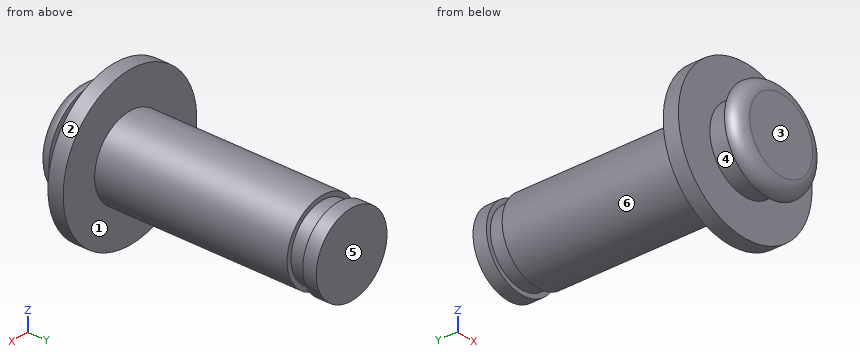
```python
from build123d import *


with BuildPart() as part:
    # Esboço1 → Revolução1 (revolve)
    with BuildSketch(Plane(origin=(0, 0, 0), x_dir=(0, 0, -1), z_dir=(1, 0, 0)), mode=Mode.PRIVATE) as revolu_o1_sk:
        with BuildLine():
            Line((0, 30.4), (0, 0))
            Line((0, 0), (-4, 0))
            ThreePointArc((-4, 0), (-5.060660172, 0.439339828), (-5.5, 1.5))
            Line((-5.5, 1.5), (-4.5, 1.5))
            Line((-4.5, 1.5), (-4.5, 4))
            Line((-4.5, 4), (-8.5, 4))
            Line((-8.5, 4), (-8.5, 5.7))
            Line((-8.5, 5.7), (-4.5, 5.7))
            Line((-4.5, 5.7), (-4.5, 27.15))
            Line((-4.5, 27.15), (-4, 27.15))
            Line((-4, 27.15), (-4, 28.9))
            Line((-4, 28.9), (-4.5, 28.9))
            Line((-4.5, 28.9), (-4.5, 30.4))
            Line((-4.5, 30.4), (0, 30.4))
        make_face()
    revolve(revolu_o1_sk.sketch.rotate(Axis((0, 0, 0), (0, 1, 0)), 180), axis=Axis((0, 0, 0), (0, 1, 0)))


solid = part.part
```
Could you check a few things on this model? Use its own coordinates, in mm. Face numbers are marked on the shaded views. A direction names the side the tool comes from. Coordinates: 2 decimals unless noted, no trailing zeros. Order: outer loops, then holes, each group sorted by start corner. A loop starts at its lowest first (then second) coordinate and runs counter-clockwise, first axis right, second up. Notation, with made-up numbers: M 68.25,89 L 124.25,89 A15 ccw 124.25,113 Z; hole C 89.5,85 d5. An arc over 180 degrees is marked long. Use a Markdown table: item, result. Add a question column.
Q1. I want a section at D-D on x = -6.5. List the corners of the cut face in (y, z) for me.
Q2. Which directions (+Z, -Z, +X, -X, +Y, -Y) give clear straight access to the entire face, cutting with the end or side of a thin tool? Please do the marked faces 1 and 2.
Q3. If I drill on L1, parallel to Y at x = -4, z = -0.5; L2, parallel to Y at x = 1, z = -7; L3, parallel to Z at x = 0.25, y = 8, over which ranges is the centre line in solid material (lowest first)?
Q4. We'd pull the mould along Y, two halves only. Please class the marked faces 3, 4, 5 and 6: pulls with the +Y half, pulls with the -Y half, needs draft (parallel to the pull), parting line crosses it, or undercut.
Q5. I want a section at A-A on x = 0. List the corners of the cut face in (y, z) for me.
Q6. I want a section at B-B on z = 0. List the corners of the cut face in (x, y) for me, then the cut area to 3 significant figures.
Q7. I want a section at C-C on y = 23. List the corners of the cut face in (x, z) for me, then the cut area to 3 significant figures.
Q8. I'm going to push flat-ended pins straight in: pin 1 (10 mm diameter, centred on x = 0.5, z = -1.5, fed in from -Y); pin 2 (1.5 mm diameter, centred on x = -5, z = -2.5, fed in from +Y); pin 3 (5 mm diameter, centred on x = 3, y = 22.5, fed in from +Z); pin 4 (6 mm diameter, centred on x = -5.5, y = 17.5, fed in from -Z). Where does each tip first touch, or does it pass through?
Checked values:
| question | item | result |
|---|---|---|
| 1 | outline | M 4,-5.48 L 5.7,-5.48 L 5.7,5.48 L 4,5.48 Z |
| 2 | face 1 | +Y |
| 2 | face 2 | +Y, -Y |
| 3 | L1 | 0 to 27.15, 28.9 to 30.4 |
| 3 | L2 | 4 to 5.7 |
| 3 | L3 | -4.49 to 4.49 |
| 4 | face 3 | pulls with the -Y half |
| 4 | face 4 | undercut |
| 4 | face 5 | pulls with the +Y half |
| 4 | face 6 | needs draft |
| 5 | outline | M 0,-4 A1.5 ccw 1.5,-5.5 L 1.5,-4.5 L 4,-4.5 L 4,-8.5 L 5.7,-8.5 L 5.7,-4.5 L 27.15,-4.5 L 27.15,-4 L 28.9,-4 L 28.9,-4.5 L 30.4,-4.5 L 30.4,4.5 L 28.9,4.5 L 28.9,4 L 27.15,4 L 27.15,4.5 L 5.7,4.5 L 5.7,8.5 L 4,8.5 L 4,4.5 L 1.5,4.5 L 1.5,5.5 A1.5 ccw 0,4 Z |
| 6 | outline | M -8.5,4 L -4.5,4 L -4.5,1.5 L -5.5,1.5 A1.5 ccw -4,0 L 4,0 A1.5 ccw 5.5,1.5 L 4.5,1.5 L 4.5,4 L 8.5,4 L 8.5,5.7 L 4.5,5.7 L 4.5,27.15 L 4,27.15 L 4,28.9 L 4.5,28.9 L 4.5,30.4 L -4.5,30.4 L -4.5,28.9 L -4,28.9 L -4,27.15 L -4.5,27.15 L -4.5,5.7 L -8.5,5.7 Z |
| 6 | area | 287 mm² |
| 7 | outline | C 0,0 d9 |
| 7 | area | 63.6 mm² |
| 8 | pin 1 | y = 0 |
| 8 | pin 2 | y = 5.7 |
| 8 | pin 3 | z = 4.47 |
| 8 | pin 4 | z = -3.74 |
